Can you work these out from the model? Positions are in its coordinate system, mm. Face numbers are marked on the shaded views. A direction names the side the tool comes from. Give positions to 0.01 mm unless a question says otherwise; leave off trailing zeros. Order: outer loops, then holes, each group sorted by start corner. A loop starts at its lowest first (then second) coordinate and runs counter-clockwise, first axis right, second up. Notation, with made-up numbers: (-13, 59) - (32, 59) arc R19 cw to (32, 82) - close; hole circle Ø11 at (-38.5, -20). An arc over 180 degrees is marked (long way). Use one line per item in the form item = value. Start each with the question number.
1) Please list where these lines run through material, in increasing order: probe 1 along Y at (x, z) = (0, 2.55) (3 decimals); probe 2 along Y at (x, z) = (2.54, 3.8) (3 decimals); probe 3 along Y at (x, z) = (0.25, 68).
2) Suppose I cut it at A-A, the plane z = 7.5. Write out the boundary of the cut face in (x, y).
3) Which directions (+Z, -Z, +X, -X, +Y, -Y) give clear straight access to the entire face, cutting with the end or side of a thin tool? Please do the marked faces 1 and 2.
4) Suppose I cut it at B-B, the plane z = 86. Write out the boundary of the cut face in (x, y), and give its area (3 significant figures).
5) For pin 1 (3 mm diameter, centred on x = -2.5, z = 47.5, fed in from +Y); pin 2 (0.6 mm diameter, centred on x = -2.5, y = 0, fed in from -Z); pin 3 (3 mm diameter, centred on x = -0.5, y = 2, fed in from -Z), each with a flat end and sliding along its axis, tell me the tip position at first contact or that it passes through.
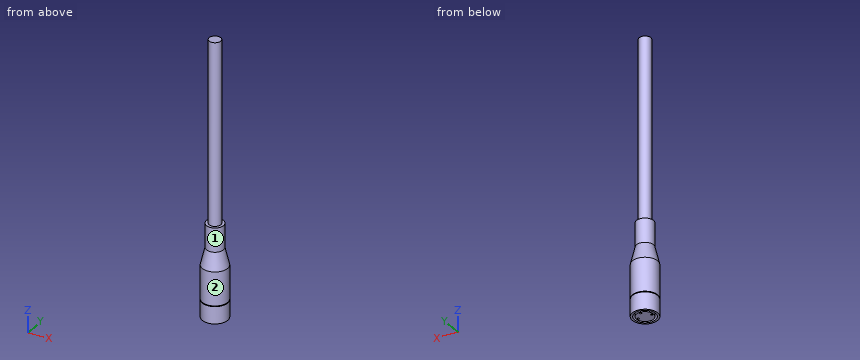
```python
from build123d import *

# Parameters (mm, degrees)
SKETCH2_R          = 2.159
EXTRUDE1_DEPTH     = 101.6
SKETCH4_R          = 3.937
SKETCH4_R_2        = 3.175
SKETCH4_R_3        = 0.381
CUT_EXTRUDE2_DEPTH = 5.08


with BuildPart() as part:
    # S2D0001 → Revolve1 (revolve)
    with BuildSketch(Plane(origin=(0, 0, 0), x_dir=(0, 0, -1), z_dir=(1, 0, 0)), mode=Mode.PRIVATE) as revolve1_sk:
        Polygon((0, 0), (0, 4.699), (-6.35, 4.699), (-6.35, 4.445), (-6.604, 4.445), (-6.604, 4.699), (-19.05, 4.699), (-25.4, 3.175), (-34.29, 3.175), (-34.29, 0), align=None)
    revolve(revolve1_sk.sketch.rotate(Axis((0, 0, 36.0045), (0, 0, -1)), 90), axis=Axis((0, 0, 36.0045), (0, 0, -1)))  # turned: the seam where the file's is

    # Sketch2 → Extrude1 (add)
    with BuildSketch(Plane(origin=(0, 0, 0), x_dir=(-1, 0, 0), z_dir=(0, 0, -1))):
        Circle(SKETCH2_R)
    extrude(amount=-EXTRUDE1_DEPTH)

    # Sketch4 → Cut-Extrude2 (cut)
    with BuildSketch(Plane(origin=(0, 0, 0), x_dir=(-1, 0, 0), z_dir=(0, 0, -1))):
        Circle(SKETCH4_R)
        with Locations(Location((0, 0, 0), (0, 0, 180))):  # turned: the seam where the file's is
            Circle(SKETCH4_R_2, mode=Mode.SUBTRACT)
        with Locations((0, 2.54)):
            Circle(SKETCH4_R_3)
        with Locations((2.54, 0)):
            Circle(SKETCH4_R_3)
        with Locations((-2.54, 0)):
            Circle(SKETCH4_R_3)
    extrude(amount=-CUT_EXTRUDE2_DEPTH, mode=Mode.SUBTRACT)


solid = part.part
```
Result sheet:
q1.probe_1 = -4.699 to -3.937, -3.175 to 2.159, 2.921 to 3.175, 3.937 to 4.699
q1.probe_2 = -3.953 to -3.008, -1.905 to -0.381, 0.381 to 1.905, 3.008 to 3.953
q1.probe_3 = -2.14 to 2.14
q2.outline = circle Ø9.4 at (0, 0)
q3.face_1 = +Z
q3.face_2 = +Z, -Z
q4.outline = circle Ø4.32 at (0, 0)
q4.area = 14.6 mm²
q5.pin_1 = 1.91
q5.pin_2 = 5.08
q5.pin_3 = 0
